from build123d import *

# Parameters (mm, degrees)
F1_DEPTH = 30
F2_R     = 1.55
F3_DEPTH = 25
F5_DEPTH = 25
F6_R     = 0.7
F7_DEPTH = 25


with BuildPart() as f1:
    # F0 (on Top) → F1 (new body)
    with BuildSketch(Plane.XY):
        with BuildLine():
            Line((3.1, 40), (0, 40))
            Line((0, 40), (-3.1, 40))
            Line((-3.1, 40), (-3.1, 21.539828))
            ThreePointArc((-3.1, 21.539828), (-3.314209, 20.092001), (-3.938482, 18.768229))
            add(Edge.make_bspline(
                [(-3.938482, 18.768229), (-5.157937, 16.937234), (-5.993951, 15.261912), (-6, 11.27962)],
                knots=[1.631065, 1.631065, 1.631065, 1.631065, 9.189941, 9.189941, 9.189941, 9.189941], degree=3))
            Line((-6, 11.27962), (-6, 0))
            Line((-6, 0), (-2, 0))
            Line((-2, 0), (-2, 15))
            Line((-2, 15), (0, 15))
            Line((0, 15), (2, 15))
            Line((2, 15), (2, 0))
            Line((2, 0), (6, 0))
            Line((6, 0), (6, 11.27962))
            add(Edge.make_bspline(
                [(3.938482, 18.768229), (5.157937, 16.937234), (5.993951, 15.261912), (6, 11.27962)],
                knots=[1.631065, 1.631065, 1.631065, 1.631065, 9.189941, 9.189941, 9.189941, 9.189941], degree=3))
            ThreePointArc((3.938482, 18.768229), (3.314209, 20.092001), (3.1, 21.539828))
            Line((3.1, 21.539828), (3.1, 40))
        make_face()
    extrude(amount=F1_DEPTH)

    # F2 (on face) → F3 (cut)
    with BuildSketch(Plane.YZ.offset(3.1)):
        with Locations((30, 22)):
            Circle(F2_R)
        with BuildLine():
            ThreePointArc((26.592245, 6.879246), (30, 6.5), (33.407755, 6.879246))
            ThreePointArc((33.407755, 6.879246), (34.541271, 8.672327), (32.74819, 9.805843))
            ThreePointArc((32.74819, 9.805843), (30, 9.5), (27.25181, 9.805843))
            ThreePointArc((27.25181, 9.805843), (25.458729, 8.672327), (26.592245, 6.879246))
        make_face()
    extrude(amount=-F3_DEPTH, mode=Mode.SUBTRACT)

    # F4 (on face) → F5 (cut)
    with BuildSketch(Plane.YZ.offset(6)):
        Polygon((3, 0), (0, 30), (0, 0), align=None)
    extrude(amount=-F5_DEPTH, mode=Mode.SUBTRACT)

    # F6 (on face) → F7 (cut)
    with BuildSketch(Plane.YZ.offset(6)):
        with Locations((8.27962, 27)):
            Circle(F6_R)
        with Locations((5.27962, 27)):
            Circle(F6_R)
        with Locations((2.27962, 27)):
            Circle(F6_R)
        with Locations((5.256872, 24.000086)):
            Circle(F6_R)
        with Locations((8.256872, 24.000086)):
            Circle(F6_R)
        with Locations((5.234124, 21.000172)):
            Circle(F6_R)
        with Locations((8.234124, 21.000172)):
            Circle(F6_R)
        with Locations((5.211376, 18.000259)):
            Circle(F6_R)
        with Locations((8.211376, 18.000259)):
            Circle(F6_R)
        with Locations((5.188628, 15.000345)):
            Circle(F6_R)
        with Locations((8.188628, 15.000345)):
            Circle(F6_R)
        with Locations((5.16588, 12.000431)):
            Circle(F6_R)
        with Locations((8.16588, 12.000431)):
            Circle(F6_R)
        with Locations((5.143132, 9.000517)):
            Circle(F6_R)
        with Locations((8.143132, 9.000517)):
            Circle(F6_R)
        with Locations((5.120384, 6.000604)):
            Circle(F6_R)
        with Locations((8.120384, 6.000604)):
            Circle(F6_R)
    extrude(amount=-F7_DEPTH, mode=Mode.SUBTRACT)


solid = f1.part
CAD build for the part. Positions are in the model's coordinates, mm. A direction names the side the tool comes from. Round coordinates to 2 decimals unless told otherwise and drop trailing zeros. Loops run counter-clockwise (first coordinate to the right, second up) from the corner with the lowest first, then second, coordinate; pieces in that order, holes last.
(1) Wall check: line 1 along Z through (x, y) = (-1.5, 30); line 2 along X through (y, z) = (2, 28); line 3 along Y through (x, z) = (3, 26.5). Give the ranges that are in metal, low to high.
(2) Cut at B-B (x = -2.5). State how many separate pieces and enclosed holes the cut face has, plus the area to 3 significant figures.
(3) Drop flat-ended pins along their axis: pin 1 (1.5 mm diameter, centred on x = 4.5, z = 20.5, fed in from -Y) (3 decimals); pin 2 (1 mm diameter, centred on y = 25, z = 19.5, fed in from +X). Give the stop position or say it passes through.
(4) Cut at C-C (y = 10). Give the cut face in (x, z).
(5) Cut at A-A (y = 30). Give the cut face in (x, z), plus the area to 3 significant figures.
(6) Two-plate mould, pull along Y, no slides. Class faces 4 (the cylindrical face through (-3.97, 4.49, 15.03)), 5 (the flat face through (-3.97, 1.52, 14.79)), 6 (the cylindrical face through (-3.31, 20.11, 14.79)): +Y half, -Y half, draft (parallel to the pull), parting line (faces both ways), or undercut.
(7) Which spindle directions (+Z, -Z, +X, -X, +Y, -Y) get a long thin tool onto all of the face, cutting with end or side? Do faces 1 (the flat face through (0, 22, 0)), 2 (the flat face through (2, 9.3, 14.8)), 3 (the cylindrical face through (0.043, 25.466, 8.704)). Say none if no direction does.
Findings below:
1. line 1: z = 0 to 6.5, 9.5 to 20.45, 23.55 to 30
1. line 2: x = -6 to -2, 2 to 6
1. line 3: y = 0.35 to 1.79, 2.77 to 4.79, 5.77 to 7.79, 8.77 to 40
2. separate pieces: 1
2. enclosed holes: 19
2. area: 1,100 mm2
3. pin 1: stops at y = 0.875
3. pin 2: stops at x = 3.1
4. outline: (-6, 0) - (-2, 0) - (-2, 30) - (-6, 30) - close; (2, 0) - (6, 0) - (6, 30) - (2, 30) - close
5. outline: (-3.1, 0) - (3.1, 0) - (3.1, 6.5) - (-3.1, 6.5) - close; (-3.1, 9.5) - (3.1, 9.5) - (3.1, 20.45) - (-3.1, 20.45) - close; (-3.1, 23.55) - (3.1, 23.55) - (3.1, 30) - (-3.1, 30) - close
5. area: 148 mm2
6. face 4: undercut
6. face 5: -Y half
6. face 6: +Y half
7. face 1: -Z, +X, -X, +Y, -Y
7. face 2: +Z, -Z, -Y
7. face 3: +X, -X
